```python
from build123d import *

# Parameters (mm, degrees)
SKETCH_W        = 43.922756
SKETCH_H        = 45
SKETCH_R        = 3.1
PAD_DEPTH       = 12
SKETCH001_W     = 26.2
SKETCH001_H     = 24.8
POCKET_DEPTH    = 10
SKETCH002_R     = 5
POCKET001_DEPTH = 1
FILLET_R        = 4
SKETCH003_W     = 16.2
SKETCH003_H     = 10
POCKET002_DEPTH = 5
FILLET001_R     = 1


with BuildPart() as part:
    # Sketch → Pad (new body)
    with BuildSketch(Plane.XY):
        with Locations((0, 9.5)):
            Rectangle(SKETCH_W, SKETCH_H)
        Circle(SKETCH_R, mode=Mode.SUBTRACT)
    extrude(amount=PAD_DEPTH)

    # Sketch001 (on Face7 of Pad) → Pocket (cut)
    with BuildSketch(Plane.XY.offset(12)):
        with Locations((0, 17.8)):
            Rectangle(SKETCH001_W, SKETCH001_H)
    extrude(amount=-POCKET_DEPTH, mode=Mode.SUBTRACT)

    # Sketch002 (on Face4 of Pocket) → Pocket001 (cut)
    with BuildSketch(Plane(origin=(0, 0, 0), x_dir=(1, 0, 0), z_dir=(0, 0, -1))):
        Circle(SKETCH002_R)
    extrude(amount=-POCKET001_DEPTH, mode=Mode.SUBTRACT)

    # Fillet
    fillet_edges = [part.edges().sort_by_distance(p)[0] for p in [
        (21.961378, 32, 6),
        (-21.961378, 32, 6),
        (21.961378, -13, 6),
        (-21.961378, -13, 6),
    ]]
    fillet(fillet_edges, radius=FILLET_R)

    # Sketch003 (on Face16 of Fillet) → Pocket002 (cut)
    with BuildSketch(Plane.XZ.offset(-30.2)):
        with Locations((0, 7)):
            Rectangle(SKETCH003_W, SKETCH003_H)
    extrude(amount=-POCKET002_DEPTH, mode=Mode.SUBTRACT)

    # Fillet001
    fillet001_edges = [part.edges().sort_by_distance(p)[0] for p in [
        (8.1, 31.1, 2),
        (-8.1, 31.1, 2),
    ]]
    fillet(fillet001_edges, radius=FILLET001_R)


solid = part.part
```
Could you check a few things on this model? Use its own coordinates, in mm. A direction names the side the tool comes from. Round coordinates to 2 decimals unless told otherwise and drop trailing zeros. Loops run counter-clockwise (first coordinate to the right, second up) from the corner with the lowest first, then second, coordinate; pieces in that order, holes last. Notation, with made-up numbers: (56.5, -30) - (79.5, -30) arc R20 cw to (79.5, -13) - close; hole circle Ø5 at (72, 36.25). An arc over 180 degrees is marked (long way). Answer in a Markdown table with one row per item. Add a question column.
(1) I'm going to push flat-ended pins straight in: pin 1 (7 mm diameter, centred on x = 0, y = 0, fed in from -Z); pin 2 (0.9 mm diameter, centred on y = 31.5, z = 5.5, fed in from -X); pin 3 (6 mm diameter, centred on x = 0, y = 0, fed in from +Z); pin 4 (0.9 mm diameter, centred on y = 30.5, z = 7, fed in from +X). Where does each tip first touch, or does it pass through?
(2) If we section it at A-A (y = 0): Please give me the cut outline in (x, z), plus the area to 3 significant figures.
(3) If we section it at B-B (x = 0): Please give me the cut outline in (y, z).
(4) If we section it at D-D (y = 18): Please give me the cut outline in (x, z), plus the area to 3 significant figures.
(5) If we mould it in two halves opening along X, with no side actions, what happens to faces 4 (the face through (-20.82, 30.8, 6.08)), 5 (the face through (0, -13, 6)), 6 (the face through (11, 30.2, 7))? For each: pulls with the +X half, pulls with the -X half, needs draft (parallel to the pull), parting line crosses it, or undercut.
(6) For faces 1 (the face through (0, 19, 2)), 2 (the face through (-1.08, 4.88, 0.49)), 3 (the face through (-7.815, 31.113, 2.301)), which set-ups out of +Z, -Z, +X, -X, +Y, -Y let a thin tool reach every point of the face, with its end or its side?
(7) I need wall thicknesses on line 1 along X through (y, z) = (5.5, 5.5); line 2 along Y through (x, z) = (0, 0.4); line 3 along X through (y, z) = (0, 6). Which ranges of each line are inside material? Lowest first, please.
(8) If we section it at C-C (z = 4): Please give me the cut outline in (x, y).
Model answer:
| question | item | result |
|---|---|---|
| 1 | pin 1 | stops at z = 1 |
| 1 | pin 2 | stops at x = -20.55 |
| 1 | pin 3 | passes through |
| 1 | pin 4 | stops at x = 21.4 |
| 2 | outline | (-21.96, 0) - (-5, 0) - (-5, 1) - (-3.1, 1) - (-3.1, 12) - (-21.96, 12) - close; (3.1, 1) - (5, 1) - (5, 0) - (21.96, 0) - (21.96, 12) - (3.1, 12) - close |
| 2 | area | 449 mm² |
| 3 | outline | (-13, 0) - (-5, 0) - (-5, 1) - (-3.1, 1) - (-3.1, 12) - (-13, 12) - close; (3.1, 1) - (5, 1) - (5, 0) - (32, 0) - (32, 2) - (5.4, 2) - (5.4, 12) - (3.1, 12) - close |
| 4 | outline | (-21.96, 0) - (21.96, 0) - (21.96, 12) - (13.1, 12) - (13.1, 2) - (-13.1, 2) - (-13.1, 12) - (-21.96, 12) - close |
| 4 | area | 265 mm² |
| 5 | face 4 | pulls with the -X half |
| 5 | face 5 | needs draft |
| 5 | face 6 | undercut |
| 6 | face 1 | +Z |
| 6 | face 2 | -Z |
| 6 | face 3 | +Z, +Y |
| 7 | line 1 | x = -21.96 to -13.1, 13.1 to 21.96 |
| 7 | line 2 | y = -13 to -5, 5 to 32 |
| 7 | line 3 | x = -21.96 to -3.1, 3.1 to 21.96 |
| 8 | outline | (-21.96, -9) arc R4 ccw to (-17.96, -13) - (17.96, -13) arc R4 ccw to (21.96, -9) - (21.96, 28) arc R4 ccw to (17.96, 32) - (8.1, 32) - (8.1, 30.2) - (13.1, 30.2) - (13.1, 5.4) - (-13.1, 5.4) - (-13.1, 30.2) - (-8.1, 30.2) - (-8.1, 32) - (-17.96, 32) arc R4 ccw to (-21.96, 28) - close; hole circle Ø6.2 at (0, 0) |
